The figure shows three views and two pictorial views of one solid part (mm, origin at its lowest corner). Answer the questions. A direction names the side the tool comes from. Coordinates: 2 decimals unless noted, no trailing zeros. Write each loop counter-clockwise with the first axis right and the second up, starting at its lowest first coordinate (ties: lowest second). Pieces come first, ordered by that corner, then holes. Notation, with made-up numbers: M 52.25,83.25 L 108.25,83.25 A22 ccw 108.25,100.25 Z; hole C 54,-30 d3. An arc over 180 degrees is marked long. Write item = value, one per line. Start each with the question number.
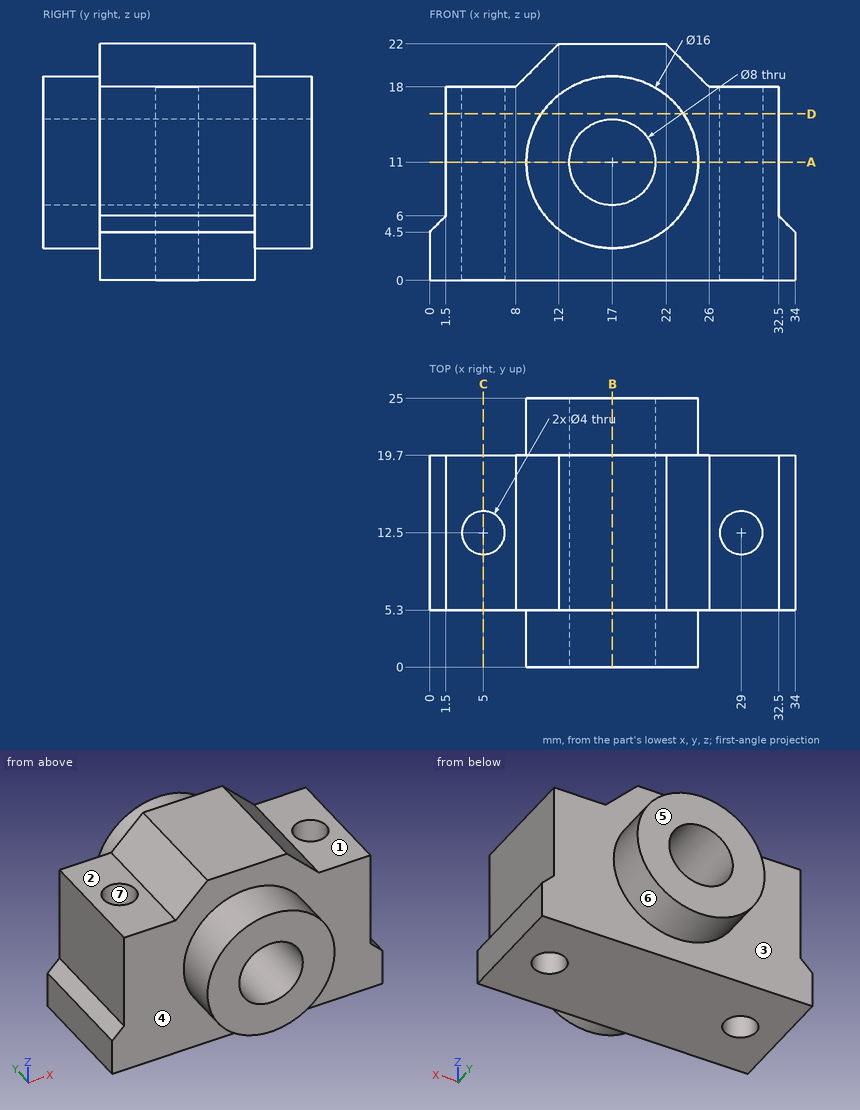
1. The part is cut by section C-C, the plane x = 5. Write down the section's boundary in (y, z), and give its area (3 significant figures).
2. Each of these flat-tipped pins is pushed along its axis until it touches: pin 1 (12 mm diameter, centred on y = 18, z = 15.5, fed in from +X); pin 2 (5 mm diameter, centred on y = 20, z = 4.5, fed in from +X); pin 3 (6.5 mm diameter, centred on x = 5, y = 12.5, fed in from +Z); pin 4 (5 mm diameter, centred on x = 4, y = 13, fed in from +Z). Where does it stop, or does it pass through?
3. Straight lines are drawn through the part: L1, parallel to Y at x = 5, z = 12; L2, parallel to Z at x = 17, y = 16.5; L3, parallel to X at y = 9.5, z = 11. For each, find the intervals that lie inside material, in ascending order. Write a range as [from, to].
4. For a pull along X with two mould halves and no side action, classify the marked faces 5, 6 and 7 as pulls with the +X half, pulls with the -X half, needs draft (parallel to the pull), parting line crosses it, or undercut.
5. The part is cut by section D-D, the plane z = 15.5. Write down the section's boundary in (x, y), and give its area (3 significant figures).
6. For the marked faces 1, 2, 3 and 4, determine the directions among +Z, -Z, +X, -X, +Y, -Y from which every point of the face is accessible in a straight line to the end or side of a thin tool.
7. The part is cut by section A-A, the plane z = 11. Write down the section's boundary in (x, y), and give its area (3 significant figures).
8. The part is cut by section B-B, the plane x = 17. Write down the section's boundary in (y, z).
Solution:
q1.outline = M 5.3,0 L 10.5,0 L 10.5,18 L 5.3,18 Z; M 14.5,0 L 19.7,0 L 19.7,18 L 14.5,18 Z
q1.area = 187 mm^2
q2.pin_1 = 32.5
q2.pin_2 = 34
q2.pin_3 = 18.25
q2.pin_4 = 18
q3.L1 = [5.3, 10.5], [14.5, 19.7]
q3.L2 = [0, 7], [15, 22]
q3.L3 = [1.5, 13], [21, 32.5]
q4.face_5 = needs draft
q4.face_6 = parting line crosses it
q4.face_7 = undercut
q5.outline = M 1.5,5.3 L 10.39,5.3 L 10.39,0 L 23.61,0 L 23.61,5.3 L 32.5,5.3 L 32.5,19.7 L 23.61,19.7 L 23.61,25 L 10.39,25 L 10.39,19.7 L 1.5,19.7 Z; hole C 5,12.5 d4; hole C 29,12.5 d4
q5.area = 561 mm^2
q6.face_1 = +Z, +X, +Y, -Y
q6.face_2 = +Z, -X, +Y, -Y
q6.face_3 = +Y
q6.face_4 = -Y
q7.outline = M 1.5,5.3 L 9,5.3 L 9,0 L 13,0 L 13,25 L 9,25 L 9,19.7 L 1.5,19.7 Z; M 21,0 L 25,0 L 25,5.3 L 32.5,5.3 L 32.5,19.7 L 25,19.7 L 25,25 L 21,25 Z; hole C 5,12.5 d4; hole C 29,12.5 d4
q7.area = 391 mm^2
q8.outline = M 0,3 L 5.3,3 L 5.3,0 L 19.7,0 L 19.7,3 L 25,3 L 25,7 L 0,7 Z; M 0,15 L 25,15 L 25,19 L 19.7,19 L 19.7,22 L 5.3,22 L 5.3,19 L 0,19 Z
